from build123d import *

# Parameters (mm, degrees)
F0_R     = 64
F1_DEPTH = 1
F2_W     = 50
F2_H     = 214.946085466
F3_DEPTH = 1
F4_R     = 10
F5_COUNT = 8
F6_R     = 10


with BuildPart() as f1:
    # F0 (on Top) → F1 (new body)
    with BuildSketch(Plane.XY):
        Circle(F0_R)
    extrude(amount=F1_DEPTH)

    # F2 (on Top) → F3 (join)
    with BuildSketch(Plane.XY):
        with Locations((0, 166.3882360196)):
            Rectangle(F2_W, F2_H)
    extrude(amount=F3_DEPTH)

    # F4
    f4_edges = [f1.edges().sort_by_distance(p)[0] for p in [
        (-25, 273.861279, 0.5),
        (25, 273.861279, 0.5),
    ]]
    fillet(f4_edges, radius=F4_R)

    # F5: F1 ×8 about axis
    f5_axis = Axis((0, 0, 0), (0, 0, 1))


with BuildPart() as f1_1:
    add(f1.part)
    for i in range(1, F5_COUNT):
        add(f1.part.rotate(f5_axis, i * 360 / F5_COUNT))

    # F6
    f6_edges = [f1_1.edges().sort_by_distance(p)[0] for p in [
        (25, -60.355339, 0.5),
        (25, 60.355339, 0.5),
        (-25, 60.355339, 0.5),
        (-25, -60.355339, 0.5),
        (60.355339, -25, 0.5),
        (60.355339, 25, 0.5),
        (-60.355339, -25, 0.5),
        (-60.355339, 25, 0.5),
    ]]
    fillet(f6_edges, radius=F6_R)


solid = f1_1.part
Source: CAD feature listing. Evaluate the final solid. Frame: model axes, mm. A direction names the side the tool comes from. Coordinates: 2 decimals unless noted, no trailing zeros. Loops run counter-clockwise (first coordinate to the right, second up) from the corner with the lowest first, then second, coordinate; pieces in that order, holes last. Notation, with made-up numbers: (23, -33.75) - (66, -33.75) arc R27 ccw to (66, -9.75) - close; hole circle Ø11 at (81, 8). An arc over 180 degrees is marked (long way). Return JSON: item names as keys, results as strings.
Q1. Section B-B, the plane x = 117.5. Return loops of the section in (y, z), plus the area to 3 significant figures.
Results:
{"outline": "(-152.86, 0) - (-82.14, 0) - (-82.14, 1) - (-152.86, 1) - close; (-25, 0) - (25, 0) - (25, 1) - (-25, 1) - close; (82.14, 0) - (152.86, 0) - (152.86, 1) - (82.14, 1) - close", "area": "191 mm2"}
Q2. Material intervals for line 1 along Y through (x, z) = (129.5, 0.45); line 2 along X through (y, z) = (199.5, 0.55); line 3 along X through (y, z) = (171, 0.4), sorted ascending.
Results:
{"line 1": "-164.86 to -94.14, -25 to 25, 94.14 to 164.86", "line 2": "-187.8 to -164.14, -25 to 25, 164.14 to 187.8", "line 3": "-205.86 to -135.64, -25 to 25, 135.64 to 205.86"}
Q3. Contact query for flat-ended pins moving along their axis: P1, Ø1.5, axis at x = 23, y = 180, coming from the -Z side; P2, Ø0.5, axis at y = -131, z = 0.5, coming from the -X side; P3, Ø0.5, axis at x = 208, z = 0.5, coming from the -Y side; P4, Ø0.5, axis at y = 209, z = 0.5, coming from the +X side. Output: stop coordinate, or through.
Results:
{"P1": "z = 0", "P2": "x = -166.61", "P3": "y = -25", "P4": "x = 25"}
Q4. Section A-A, the plane y = 196. Return loops of the section in (x, z), plus the area to 3 significant figures.
Results:
{"outline": "(-191.3, 0) - (-160.64, 0) - (-160.64, 1) - (-191.3, 1) - close; (-25, 0) - (25, 0) - (25, 1) - (-25, 1) - close; (160.64, 0) - (191.3, 0) - (191.3, 1) - (160.64, 1) - close", "area": "111 mm2"}
Q5. Access query for faces 1 (the flat face through (-104.598, 139.953, 0.493)), 2 (the flat face through (104.598, -139.953, 0.493)), 3 (the flat face through (-139.953, 104.598, 0.493)). Directions: +Z, -Z, +X, -X, +Y, -Y. A direction counts if a zero-diameter tool reaches every point of the face in a straight line with its end or side. Return the directions, or none.
Results:
{"face 1": "+Z, -Z, +Y", "face 2": "+Z, -Z, -Y", "face 3": "+Z, -Z, -X"}
Q6. Section C-C, the plane x = -64. Return loops of the section in (y, z), plus the area to 3 significant figures.
Results:
{"outline": "(-99.36, 0) - (99.36, 0) - (99.36, 1) - (-99.36, 1) - close", "area": "199 mm2"}
Q7. Mould query, pull axis Y, two halves, no side actions, for faces 4 (the flat face through (139.953, 104.598, 0.493)), 5 (the flat face through (-139.953, -104.598, 0.493)), 6 (the flat face through (-104.598, -139.953, 0.493)), 7 (the flat face through (1, -19, 0)). Classes: released by +Y, released by -Y, zero draft, split by the parting line, or undercut.
Results:
{"face 4": "undercut", "face 5": "undercut", "face 6": "released by -Y", "face 7": "zero draft"}
